Autodesk Inventor part; units mm, degrees
ref_plane "YZ Plane" through (0, 0, 0) normal (1, 0, 0) x (0, 1, 0)
ref_plane "XZ Plane" through (0, 0, 0) normal (0, 1, 0) x (-1, 0, 0)
ref_plane "XY Plane" through (0, 0, 0) normal (0, 0, 1) x (1, 0, 0)
sketch "Sketch1" plane through (0, 0, 0) normal (0, 0, 1) x (1, 0, 0)
  line L0 (0, -16.2697) -> (0, 26.8303)
  line L1 (0, -16.2697) -> (10.125, -16.2697)
  line L2 (10.125, -16.2697) -> (10.125, -11.5997)
  line L3 (10.125, -11.5997) -> (12.15, -11.5997)
  line L4 (12.15, -11.5997) -> (12.15, -2.3297)
  line L5 (12.15, -2.3297) -> (10.125, -2.3297)
  line L6 (8.1117, 22.1005) -> (7.73, 23.0903)
  line L7 (7.73, 23.0903) -> (2.4142, 25.6622)
  line L8 (2.5391, 25.6018) -> (2.4142, 25.6622)
  line L9 (0, 31.6595) -> (0, 26.8303)
  line L10 (0, 31.6595) -> (0.4457, 31.6595)
  line L11 (0.4457, 31.6595) -> (2.4142, 25.6622)
  line L12 (10.125, -2.3297) -> (10.125, 2.6703)
  line L13 (10.125, 2.6703) -> (8.1117, 2.6703)
  line L14 (8.1117, 2.6703) -> (8.1117, 22.1005)
  point P0 (0, 0)
  point P1 (10.125, 16.8803)
  dimension "d0" = 43.1
  dimension "d1" = 10.125
  dimension "d2" = 4.67
  dimension "d3" = 2.025
  dimension "d4" = 90
  dimension "d5" = 9.27
  dimension "d8" = 39.36
  dimension "d10" = 5
revolve "Revolution1" add sketch "Sketch1" angle 360 about axis through (0, -16.2697, 0) along (0, 1, 0)
properties part number "00_objectivelens_10x"
Geometry: final body of the model. Coordinates: model frame, mm. A direction names the side the tool comes from. Round coordinates to 2 decimals unless told otherwise and drop trailing zeros. Loops run counter-clockwise (first coordinate to the right, second up) from the corner with the lowest first, then second, coordinate; pieces in that order, holes last.
Item 1: Contact query for flat-ended pins moving along their axis: P1, Ø4, axis at x = -8, y = 16.5, coming from the +Z side; P2, Ø1.5, axis at x = 2.5, y = 14, coming from the -Z side; P3, Ø10, axis at x = 7, z = -7, coming from the +Y side. Output: stop coordinate, or through.
Checked values:
P1: stops at z = 5.46
P2: stops at z = -7.92
P3: stops at y = 24.46
Item 2: Line query: L1, parallel to Y at x = -1.5, z = 8.5; L2, parallel to X at y = 20, z = 0. Output: solid intervals per line, ascending.
Checked values:
L1: y = -16.27 to 2.67
L2: x = -8.11 to 8.11
Item 3: Section A-A, the plane y = 7.5. Output: boundary loops of the cut face in (x, z), plus the area to 3 significant figures.
Checked values:
outline: circle Ø16.22 at (0, 0)
area: 207 mm2
Item 4: Section B-B, the plane y = -9. Output: boundary loops of the cut face in (x, z), plus the area to 3 significant figures.
Checked values:
outline: circle Ø24.3 at (0, 0)
area: 464 mm2
Item 5: Reachability of faces 1 (the cylindrical face through (-5.98, 12.52, -5.48)), 2 (the flat face through (-5, -11.6, -9)), 3 (the flat face through (0, -16.27, 0)) from +Z, -Z, +X, -X, +Y, -Y: full face, straight path, thin tool, end or side. Return the list, or none.
Checked values:
face 1: +Y
face 2: -Y
face 3: +Z, -Z, +X, -X, -Y
